from build123d import *

# Parameters (mm, degrees)
SKETCH1_R           = 1.7
BOSS_EXTRUDE1_DEPTH = 10
SKETCH2_R           = 1.4
CUT_EXTRUDE1_DEPTH  = 16
CHAMFER1_SIZE       = 1.6
CHAMFER2_SIZE       = 1.2


with BuildPart() as part:
    # Sketch1 → Boss-Extrude1 (new body)
    with BuildSketch(Plane.XY):
        Polygon((8.660254038, 0), (4.330127019, 7.5), (-4.330127019, 7.5), (-8.660254038, 0), (-4.330127019, -7.5), (4.330127019, -7.5), align=None)
        Circle(SKETCH1_R, mode=Mode.SUBTRACT)
    extrude(amount=BOSS_EXTRUDE1_DEPTH)

    # Sketch2 → Cut-Extrude1 (cut, through all)
    with BuildSketch(Plane.XZ.offset(7.5)):
        with Locations((0, 5)):
            Circle(SKETCH2_R)
    extrude(amount=-CUT_EXTRUDE1_DEPTH, mode=Mode.SUBTRACT)

    # Chamfer1
    chamfer1_edges = [part.edges().sort_by_distance(p)[0] for p in [
        (0, 7.5, 10),
        (-6.495190528, 3.75, 10),
        (-6.495190528, -3.75, 10),
        (0, -7.5, 10),
        (6.495190528, -3.75, 10),
        (6.495190528, 3.75, 10),
    ]]
    chamfer(chamfer1_edges, length=CHAMFER1_SIZE)

    # Chamfer2
    chamfer2_edges = [part.edges().sort_by_distance(p)[0] for p in [
        (0, -7.5, 0),
        (-6.495190528, -3.75, 0),
        (-6.495190528, 3.75, 0),
        (0, 7.5, 0),
        (6.495190528, 3.75, 0),
        (6.495190528, -3.75, 0),
    ]]
    chamfer(chamfer2_edges, length=CHAMFER2_SIZE)


solid = part.part
Verification items for the finished model (mm, model axes). Give positions to 0.01 mm unless a question says otherwise; leave off trailing zeros. Write each loop counter-clockwise with the first axis right and the second up, starting at its lowest first coordinate (ties: lowest second). Pieces come first, ordered by that corner, then holes. Notation, with made-up numbers: M -11.5,21.25 L 29.5,21.25 A21 ccw 29.5,45.25 Z; hole C 68.25,-30.75 d11. An arc over 180 degrees is marked long. Put each result on its own line as item: value. Start each with the question number.
1. Section check B-B (x = 0). Record the cut outline in (y, z).
2. Scan lines: line 1 along Z through (x, y) = (0, -4.75); line 2 along X through (y, z) = (-2, 4.5); line 3 along X through (y, z) = (1.5, 2). Record each from-to range of solid material in increasing order. Write a range as [from, to].
3. Draft check along X on faces 1 (the face through (1.57, -0.65, 4.93)), 2 (the face through (6, 3.39, 0.59)), 3 (the face through (-6.465, 3.802, 4.75)), 4 (the face through (-1.4, -4.28, 5.06)). Enter one of: +X half, -X half, draft (parallel to the pull), parting line (faces both ways), or undercut.
4. Go/stop test with flat-tipped pins: pin 1 Ø1.7 at (x, z) = (0, 5) entering from +Y; pin 2 Ø4 at (y, z) = (5.5, 3) entering from -X. Record where each tip stops, or that it passes through.
5. Section check C-C (z = 2.5). Record the cut outline in (x, y).
6. Section check A-A (z = 5). Record the cut outline in (x, y).
7. Section check D-D (y = -2). Record the cut outline in (x, z).
Answer list:
1. outline: M -7.5,1.2 L -6.3,0 L -1.7,0 L -1.7,3.6 L -7.5,3.6 Z; M -7.5,6.4 L -1.7,6.4 L -1.7,10 L -5.9,10 L -7.5,8.4 Z; M 1.7,0 L 6.3,0 L 7.5,1.2 L 7.5,3.6 L 1.7,3.6 Z; M 1.7,6.4 L 7.5,6.4 L 7.5,8.4 L 5.9,10 L 1.7,10 Z
2. line 1: [0, 3.6], [6.4, 10]
2. line 2: [-7.51, -1.31], [1.31, 7.51]
2. line 3: [-7.79, -0.8], [0.8, 7.79]
3. face 1: undercut
3. face 2: +X half
3. face 3: -X half
3. face 4: undercut
4. pin 1: through
4. pin 2: x = -6.64
5. outline: M -8.66,0 L -4.33,-7.5 L 4.33,-7.5 L 8.66,0 L 4.33,7.5 L -4.33,7.5 Z; hole C 0,0 d3.4
6. outline: M -8.66,0 L -4.33,-7.5 L -1.4,-7.5 L -1.4,-0.96 A1.7 cw -1.4,0.96 L -1.4,7.5 L -4.33,7.5 Z; M 1.4,-7.5 L 4.33,-7.5 L 8.66,0 L 4.33,7.5 L 1.4,7.5 L 1.4,0.96 A1.7 cw 1.4,-0.96 Z
7. outline: M -7.51,1.2 L -6.12,0 L 6.12,0 L 7.51,1.2 L 7.51,8.4 L 5.66,10 L -5.66,10 L -7.51,8.4 Z; hole C 0,5 d2.8
